The listing builds one solid part. Answer for the finished solid, in the listing's coordinates (mm). A direction names the side the tool comes from. Coordinates: 2 decimals unless noted, no trailing zeros. Write each loop counter-clockwise with the first axis right and the second up, starting at its lowest first coordinate (ties: lowest second). Pieces come first, ordered by that corner, then holes. Notation, with made-up numbers: M -35.75,36.25 L 10.25,36.25 A16 cw 10.25,46.25 Z; hole C -11.75,41 d6. An arc over 180 degrees is marked long. Put each result on its own line as item: value. Start each with the question number.
```python
from build123d import *

# Parameters (mm, degrees)
BOARD_DEPTH  = 0.6
CUT_DEPTH    = 60.97307864
HOLESSKE_R   = 0.5
HOLESSKE_R_2 = 1
HOLES_DEPTH  = 60.97307864
HOLES2SKE_R  = 0.8
HOLES2_DEPTH = 60.97307864


with BuildPart() as part:
    # BoardSke → Board (new body)
    with BuildSketch(Plane.XY):
        with BuildLine():
            Line((42.5, 4.330127019), (-17.5, 38.97114317))
            ThreePointArc((-17.5, 38.97114317), (-22.5, 38.97114317), (-25, 34.641016151))
            Line((-25, 34.641016151), (-25, -34.641016151))
            ThreePointArc((-25, -34.641016151), (-22.5, -38.97114317), (-17.5, -38.97114317))
            Line((-17.5, -38.97114317), (42.5, -4.330127019))
            ThreePointArc((42.5, -4.330127019), (45, 0), (42.5, 4.330127019))
        make_face()
    extrude(amount=BOARD_DEPTH)

    # CutSke → Cut (cut, through all)
    with BuildSketch(Plane.XY.offset(0.6)):
        with BuildLine():
            Line((31.07179677, 3), (9.16515139, 3))
            ThreePointArc((9.16515139, 3), (8.617428832, 3.163339973), (8.248636251, 3.6))
            ThreePointArc((8.248636251, 3.6), (4.5, 7.794228634), (-1.006626672, 8.94352854))
            ThreePointArc((-1.006626672, 8.94352854), (-1.569181638, 9.044582271), (-1.984499484, 9.437253933))
            Line((-1.984499484, 9.437253933), (-12.937822174, 28.408965344))
            ThreePointArc((-12.937822174, 28.408965344), (-12.778903551, 29.616072125), (-11.57179677, 29.774990748))
            Line((-11.57179677, 29.774990748), (31.57179677, 4.866025404))
            ThreePointArc((31.57179677, 4.866025404), (32.037722596, 3.741180955), (31.07179677, 3))
        make_face()
        with BuildLine():
            Line((31.07179677, -3), (9.16515139, -3))
            ThreePointArc((9.16515139, -3), (8.617428832, -3.163339973), (8.248636251, -3.6))
            ThreePointArc((8.248636251, -3.6), (4.5, -7.794228634), (-1.006626672, -8.94352854))
            ThreePointArc((-1.006626672, -8.94352854), (-1.569181638, -9.044582271), (-1.984499484, -9.437253933))
            Line((-1.984499484, -9.437253933), (-12.937822174, -28.408965344))
            ThreePointArc((-12.937822174, -28.408965344), (-12.778903551, -29.616072125), (-11.57179677, -29.774990748))
            Line((-11.57179677, -29.774990748), (31.57179677, -4.866025404))
            ThreePointArc((31.57179677, -4.866025404), (32.037722596, -3.741180955), (31.07179677, -3))
        make_face()
        with BuildLine():
            Line((-18.133974596, -25.408965344), (-7.180651906, -6.437253933))
            ThreePointArc((-7.180651906, -6.437253933), (-7.048247194, -5.881242297), (-7.242009579, -5.34352854))
            ThreePointArc((-7.242009579, -5.34352854), (-9, 0), (-7.242009579, 5.34352854))
            ThreePointArc((-7.242009579, 5.34352854), (-7.048247194, 5.881242297), (-7.180651906, 6.437253933))
            Line((-7.180651906, 6.437253933), (-18.133974596, 25.408965344))
            ThreePointArc((-18.133974596, 25.408965344), (-19.258819045, 25.87489117), (-20, 24.908965344))
            Line((-20, 24.908965344), (-20, -24.908965344))
            ThreePointArc((-20, -24.908965344), (-19.258819045, -25.87489117), (-18.133974596, -25.408965344))
        make_face()
    extrude(amount=-CUT_DEPTH, mode=Mode.SUBTRACT)

    # HolesSke → Holes (cut, through all)
    with BuildSketch(Plane.XY.offset(0.6)):
        with Locations((-6, 0)):
            Circle(HOLESSKE_R)
        with Locations((3, 5.196152423)):
            Circle(HOLESSKE_R)
        with Locations((3, -5.196152423)):
            Circle(HOLESSKE_R)
        Circle(HOLESSKE_R_2)
    extrude(amount=-HOLES_DEPTH, mode=Mode.SUBTRACT)

    # Holes2Ske → Holes2 (cut, through all)
    with BuildSketch(Plane.XY.offset(0.6)):
        with Locations((40, 0)):
            Circle(HOLES2SKE_R)
        with Locations((-20, -34.641016151)):
            Circle(HOLES2SKE_R)
        with Locations((-20, 34.641016151)):
            Circle(HOLES2SKE_R)
    extrude(amount=-HOLES2_DEPTH, mode=Mode.SUBTRACT)


solid = part.part
```
1) For faces 1 (the face through (2, 1, 0.6)), 2 (the face through (-7.384, 18.79, 0.304)), determine the directions among +Z, -Z, +X, -X, +Y, -Y from which every point of the face is accessible in a straight line to the end or side of a thin tool.
2) A cutting plane is placed at A-A on x = 0. Write down the section's boundary in (y, z), then the cut area to 3 significant figures.
3) Determine the mould class of faces 3 (the face through (45, -0.1, 0.3)), 4 (the face through (2, 1, 0)), 5 (the face through (-12.58, 15.79, 0.3)), 6 (the face through (-22.563, -38.934, 0.296)) for opening direction X: +X half, -X half, draft (parallel to the pull), parting line (faces both ways), or undercut.
4) A cutting plane is placed at B-B on y = -8. Write down the section's boundary in (x, z).
5) A cutting plane is placed at C-C on x = 19.5. Write down the section's boundary in (y, z).
6) Straight lines are drawn through the part: probe 1 along Y at (x, z) = (6.5, 0.1); probe 2 along Y at (x, z) = (21, 0.3); probe 3 along X at (y, z) = (-4, 0.3). For each, find the intervals that lie inside material, in ascending order.
7) A cutting plane is placed at D-D on z = 0.3. State how many separate pieces and enclosed holes the cut face has, then the cut area to 3 significant figures.
Answers follow:
1. face 1: +Z, +X, -X, +Y, -Y
1. face 2: +Z, -Z
2. outline: M -28.87,0 L -23.09,0 L -23.09,0.6 L -28.87,0.6 Z; M -9,0 L -1,0 L -1,0.6 L -9,0.6 Z; M 1,0 L 9,0 L 9,0.6 L 1,0.6 Z; M 23.09,0 L 28.87,0 L 28.87,0.6 L 23.09,0.6 Z
2. area: 16.5 mm²
3. face 3: +X half
3. face 4: draft
3. face 5: undercut
3. face 6: parting line
4. outline: M -25,0 L -20,0 L -20,0.6 L -25,0.6 Z; M -8.08,0 L 4.12,0 L 4.12,0.6 L -8.08,0.6 Z; M 26.14,0 L 36.14,0 L 36.14,0.6 L 26.14,0.6 Z
5. outline: M -17.61,0 L -11.84,0 L -11.84,0.6 L -17.61,0.6 Z; M -3,0 L 3,0 L 3,0.6 L -3,0.6 Z; M 11.84,0 L 17.61,0 L 17.61,0.6 L 11.84,0.6 Z
6. probe 1: y = -25.11 to -19.34, -6.22 to 6.22, 19.34 to 25.11
6. probe 2: y = -16.74 to -10.97, -3 to 3, 10.97 to 16.74
6. probe 3: x = -25 to -20, -8.06 to 8.06, 32.07 to 43
7. separate pieces: 1
7. enclosed holes: 10
7. area: 1,890 mm²
